```python
from build123d import *

# Parameters (mm, degrees)
SKETCH1_R                = 2.5
BOSS_EXTRUDE1_DEPTH      = 36
BOSS_EXTRUDE1_DEPTH_BACK = 11
CSK1_AT_2_COUNT          = 2
CSK1_AT_2_PITCH          = 25
SKETCH4_W                = 15.666666667
SKETCH4_H                = 10
CUT_EXTRUDE1_DEPTH       = 11.5


with BuildPart() as part:
    # Sketch1 → Boss-Extrude1 (new body, two sides)
    with BuildSketch(Plane(origin=(0, 0, 0), x_dir=(0, 0, -1), z_dir=(1, 0, 0))) as boss_extrude1_sk:
        with BuildLine():
            Line((-10.5, 0.5), (-10.5, 0))
            Line((-10.5, 0), (7.2, 0))
            Line((7.2, 0), (7.2, 3.5))
            Line((7.2, 3.5), (-5.621475633, 3.5))
            ThreePointArc((-5.621475633, 3.5), (-5.785558164, 3.585645625), (-5.809111186, 3.769230769))
            ThreePointArc((-5.809111186, 3.769230769), (-13.358859374, 9.602063271), (-10.5, 0.5))
        make_face()
        with Locations((-10.5, 5.5)):
            Circle(SKETCH1_R, mode=Mode.SUBTRACT)
    extrude(amount=BOSS_EXTRUDE1_DEPTH)
    extrude(boss_extrude1_sk.sketch, amount=-BOSS_EXTRUDE1_DEPTH_BACK)

    # Sketch2 → CSK1 (revolve, cut)
    with BuildSketch(Plane(origin=(0, 3.5, 0), x_dir=(0, 0, 1), z_dir=(1, 0, 0))):
        Polygon((0, 0), (0, 3.5), (2.75, 3.5), (2.75, 2.75), (5.5, 0), align=None)
    csk1 = revolve(axis=Axis((0, 9.85, 0), (0, -1, 0)), mode=Mode.SUBTRACT)

    # CSK1 at 2: CSK1 ×2
    with Locations(*[(i * CSK1_AT_2_PITCH, 0, 0) for i in range(1, CSK1_AT_2_COUNT)]):
        add(csk1, mode=Mode.SUBTRACT)

    # Sketch4 → Cut-Extrude1 (cut, through all)
    with BuildSketch(Plane(origin=(0, 0, 0), x_dir=(1, 0, 0), z_dir=(0, 1, 0))):
        with Locations((-3.166666666, -10.5)):
            Rectangle(SKETCH4_W, SKETCH4_H)
        with Locations((28.166666666, -10.5)):
            Rectangle(SKETCH4_W, SKETCH4_H)
    extrude(amount=CUT_EXTRUDE1_DEPTH, mode=Mode.SUBTRACT)


solid = part.part
```
The listing builds one solid part. Answer for the finished solid, in the listing's coordinates (mm). A direction names the side the tool comes from. Give positions to 0.01 mm unless a question says otherwise; leave off trailing zeros. Order: outer loops, then holes, each group sorted by start corner. A loop starts at its lowest first (then second) coordinate and runs counter-clockwise, first axis right, second up. Notation, with made-up numbers: (-25, -25) -> (9, -25) arc R34 cw to (9, 9) -> close; hole circle Ø10 at (17.5, -38). An arc over 180 degrees is marked (long way). Answer as CSV lines item,"result". Start each with the question number.
Q1. Given pin 1 (6.5 mm diameter, centred on x = 0, z = 0, fed in from +Y); pin 2 (1 mm diameter, centred on x = -1.5, y = 1, fed in from +Z); pin 3 (3.5 mm diameter, centred on x = 25, z = 0, fed in from +Y); pin 4 (6 mm diameter, centred on y = 5.5, z = 10.5, fed in from -X), each flat-ended and moving along its own axis, determine where each tip first touches the part or whether it passes through.
Q2. A cutting plane is placed at A-A (y = 5.5). Determine the outline of the cut face in (x, z), then the cut area to 3 significant figures.
Q3. A cutting plane is placed at B-B (z = 0). Determine the outline of the cut face in (x, y), then the cut area to 3 significant figures.
Q4. Find the intervals of material crossed by L1, parallel to Z at x = 16, y = 5.5; L2, parallel to X at y = 0.45, z = 0; L3, parallel to Z at x = 25, y = 0.6, in increasing order.
Q5. Which of the six approach directions +Z, -Z, +X, -X, +Y, -Y give full straight-line access (tool end or side, diameter ignored) to faces 1 (the flat face through (-3, 2, 5.5)), 2 (the flat face through (28, 2, 5.5)), 3 (the cylindrical face through (12.39, 7.19, 12.34))?
Q6. A cutting plane is placed at D-D (x = 32.5). Determine the outline of the cut face in (y, z).
Q7. Determine the mould class of faces 4 (the conical face through (2.85, 0.92, -0.63)), 5 (the flat face through (20.333, 4, 8)), 6 (the flat face through (13, 2, -7.2)) for opening direction Z: pulls with the +Z half, pulls with the -Z half, needs draft (parallel to the pull), parting line crosses it, or undercut.
Q8. A cutting plane is placed at C-C (x = 16). Determine the outline of the cut face in (y, z), then the cut area to 3 significant figures.
Results found:
1,pin 1,"y = 1.25"
1,pin 2,"z = 5.5"
1,pin 3,"through"
1,pin 4,"x = 4.67"
2,outline,"(4.67, 5.5) -> (20.33, 5.5) -> (20.33, 8) -> (4.67, 8) -> close; (4.67, 13) -> (20.33, 13) -> (20.33, 15.5) -> (4.67, 15.5) -> close"
2,area,"78.3 mm2"
3,outline,"(-11, 0) -> (-2.75, 0) -> (-2.75, 0.75) -> (-5.5, 3.5) -> (-11, 3.5) -> close; (2.75, 0) -> (22.25, 0) -> (22.25, 0.75) -> (19.5, 3.5) -> (5.5, 3.5) -> (2.75, 0.75) -> close; (27.75, 0) -> (36, 0) -> (36, 3.5) -> (30.5, 3.5) -> (27.75, 0.75) -> close"
3,area,"111 mm2"
4,L1,"5.5 to 8, 13 to 15.5"
4,L2,"-11 to -2.75, 2.75 to 22.25, 27.75 to 36"
4,L3,"-7.2 to -2.75, 2.75 to 5.5"
5,face 1,"+Z, -X, +Y, -Y"
5,face 2,"+Z, +X, +Y, -Y"
5,face 3,"+X, -X"
6,outline,"(0, -7.2) -> (3.5, -7.2) -> (3.5, 5.5) -> (0, 5.5) -> close"
7,face 4,"undercut"
7,face 5,"needs draft"
7,face 6,"pulls with the -Z half"
8,outline,"(0, -7.2) -> (3.5, -7.2) -> (3.5, 5.62) arc R0.2 cw to (3.77, 5.81) arc R5 ccw (long way) to (0.5, 10.5) -> (0, 10.5) -> close; hole circle Ø5 at (5.5, 10.5)"
8,area,"111 mm2"
